The listing builds one solid part. Answer for the finished solid, in the listing's coordinates (mm). Face numbers are marked on the shaded views. A direction names the side the tool comes from. Give positions to 0.01 mm unless a question says otherwise; leave off trailing zeros. Order: outer loops, then holes, each group sorted by start corner. A loop starts at its lowest first (then second) coordinate and runs counter-clockwise, first axis right, second up. Notation, with made-up numbers: (25, 34) - (34, 34) arc R18 cw to (34, 65) - close; hole circle Ø2 at (46.5, -33). An arc over 180 degrees is marked (long way). Use a Markdown table: item, result. Add a question column.
1) Flat-ended cylindrical pins translate along their axes: pin 1 (8 mm diameter, centred on y = 21, z = 7, fed in from +X); pin 2 (6 mm diameter, centred on x = 57, z = -2.5, fed in from -Y); pin 3 (10 mm diameter, centred on x = -155, z = 0.5, fed in from +Y). Find the tip coordinate at first contact, or state that the pin passes through.
2) For the marked faces 1, 2 and 3, determine the directions among +Z, -Z, +X, -X, +Y, -Y from which every point of the face is accessible in a straight line to the end or side of a thin tool.
3) Find section C-C, the plane x = 70. Determine the outline of the cut face in (y, z), plus the area to 3 significant figures.
4) Find section A-A, the plane y = 0. Determine the outline of the cut face in (x, z), plus the area to 3 significant figures.
5) Find section B-B, the plane z = 5.5. Determine the outline of the cut face in (x, y).
6) Straight lines are drawn through the part: line 1 (X direction, y = 4, z = -7); line 2 (X direction, y = -20, z = 7.5); line 3 (Z direction, x = -72.5, y = -4). For each, find the intervals that lie inside material, in ascending order.
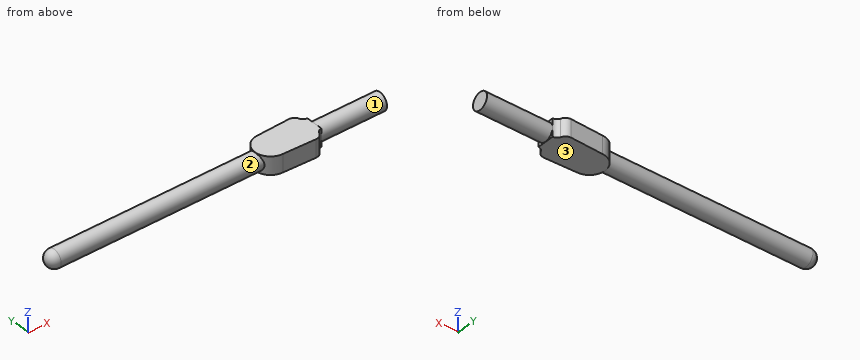
from build123d import *

# Parameters (mm, degrees)
SALIENTE_EXTRUIR1_DEPTH = 16


with BuildPart() as part:
    # Croquis1 → Revolución1 (revolve)
    with BuildSketch(Plane.XY):
        with BuildLine():
            Line((-300, 0), (300, 0))
            Line((300, 0), (300, 15.5))
            Line((300, 15.5), (-284.5, 15.5))
            ThreePointArc((-284.5, 15.5), (-295.460155108, 10.960155108), (-300, 0))
        make_face()
    revolve(axis=Axis((-657.792003839, 0, 0), (1, 0, 0)))

    # Croquis3 → Saliente-Extruir1 (add, symmetric)
    with BuildSketch(Plane.XY):
        with BuildLine():
            ThreePointArc((103.5, 28), (78.822074641, 13.228756555), (80.181552367, -15.5))
            Line((80.181552367, -15.5), (182.5, -15.5))
            Line((182.5, -15.5), (182.5, 15.5))
            ThreePointArc((182.5, 15.5), (176.96634932, 17.170611658), (173.281614908, 21.624257969))
            ThreePointArc((173.281614908, 21.624257969), (168.527455009, 27.876978724), (161.039643366, 30.25))
            Line((161.039643366, 30.25), (103.5, 28))
        make_face()
        with BuildLine():
            ThreePointArc((80.181552367, -15.5), (90.271243445, -24.677925359), (103.5, -28))
            Line((103.5, -28), (161.039643366, -30.25))
            ThreePointArc((161.039643366, -30.25), (168.527455009, -27.876978724), (173.281614908, -21.624257969))
            ThreePointArc((173.281614908, -21.624257969), (176.96634932, -17.170611658), (182.5, -15.5))
            Line((182.5, -15.5), (80.181552367, -15.5))
        make_face()
    extrude(amount=SALIENTE_EXTRUIR1_DEPTH, both=True)


solid = part.part
The answers:
| question | item | result |
|---|---|---|
| 1 | pin 1 | x = 177.23 |
| 1 | pin 2 | y = -15.5 |
| 1 | pin 3 | y = 15.5 |
| 2 | face 1 | +X |
| 2 | face 2 | -X |
| 2 | face 3 | -Z, +X, -X, +Y, -Y |
| 3 | outline | circle Ø31 at (0, 0) |
| 3 | area | 755 mm2 |
| 4 | outline | (-284.5, -15.5) - (75.5, -15.5) - (75.5, -16) - (182.5, -16) - (182.5, -15.5) - (300, -15.5) - (300, 15.5) - (182.5, 15.5) - (182.5, 16) - (75.5, 16) - (75.5, 15.5) - (-284.5, 15.5) arc R15.5 ccw to start |
| 4 | area | 18,600 mm2 |
| 5 | outline | (-284.5, -14.49) - (79.54, -14.49) arc R28 ccw to (103.5, -28) - (161.04, -30.25) arc R13 ccw to (173.28, -21.62) arc R10 cw to (182.5, -15.5) - (182.5, -14.49) - (300, -14.49) - (300, 14.49) - (182.5, 14.49) - (182.5, 15.5) arc R10 cw to (173.28, 21.62) arc R13 ccw to (161.04, 30.25) - (103.5, 28) arc R28 ccw to (79.54, 14.49) - (-284.5, 14.49) arc R14.49 ccw to start |
| 6 | line 1 | -297.74 to 300 |
| 6 | line 2 | 83.9 to 174.15 |
| 6 | line 3 | -14.97 to 14.97 |
